The model under review builds one solid part; all positions refer to its coordinate system, in mm. Round coordinates to 2 decimals unless told otherwise and drop trailing zeros. Loops run counter-clockwise (first coordinate to the right, second up) from the corner with the lowest first, then second, coordinate; pieces in that order, holes last. Notation, with made-up numbers: (1.5, -29) - (22.5, -29) arc R29 ccw to (22.5, 5) - close; hole circle Ø5 at (31.25, 65). An arc over 180 degrees is marked (long way). Answer as CSV lines item,"result".
from build123d import *

# Parameters (mm, degrees)
SKETCH1_W                     = 160
SKETCH1_H                     = 100
BASEPLATE_160X100X6_DEPTH     = 6
CORNER_FILLET_R5_R            = 5
M4_ISOLATOR_CLEARANCE_HOLES_D = 4.5


with BuildPart() as part:
    # Sketch1 → BasePlate_160x100x6 (new body)
    with BuildSketch(Plane(origin=(0, 0, 0), x_dir=(1, 0, 0), z_dir=(0, 1, 0))):
        Rectangle(SKETCH1_W, SKETCH1_H)
    extrude(amount=BASEPLATE_160X100X6_DEPTH)

    # Corner_Fillet_R5
    corner_fillet_r5_edges = [part.edges().sort_by_distance(p)[0] for p in [
        (-80, 3, -50),
        (80, 3, -50),
        (80, 3, 50),
        (-80, 3, 50),
    ]]
    fillet(corner_fillet_r5_edges, radius=CORNER_FILLET_R5_R)

    # M4_Isolator_Clearance_Holes (through all)
    with Locations(Plane(origin=(0, 6, 0), x_dir=(1, 0, 0), z_dir=(0, 1, 0))):
        with Locations((-60, 35), (60, 35), (60, -35), (-60, -35)):
            Hole(M4_ISOLATOR_CLEARANCE_HOLES_D / 2)


solid = part.part
1. Draft analysis for pull direction Z (two halves, no side actions). For faces 1 (the face through (61.66, 2.96, -36.52)), 2 (the face through (-80, 3, 1)), 3 (the face through (-79, 3, 48)), state which applies: +Z half, -Z half, draft (parallel to the pull), parting line (faces both ways), or undercut.
Numbers:
face 1,"undercut"
face 2,"draft"
face 3,"+Z half"
2. Take a section at B-B (x = 60). State the section outline as (y, z) points, plus the area to 3 significant figures.
Numbers:
outline,"(0, -50) - (6, -50) - (6, -37.25) - (0, -37.25) - close; (0, -32.75) - (6, -32.75) - (6, 32.75) - (0, 32.75) - close; (0, 37.25) - (6, 37.25) - (6, 50) - (0, 50) - close"
area,"546 mm²"
3. Take a section at A-A (z = -35). State the section outline as (x, y) points, plus the area to 3 significant figures.
Numbers:
outline,"(-80, 0) - (-62.25, 0) - (-62.25, 6) - (-80, 6) - close; (-57.75, 0) - (57.75, 0) - (57.75, 6) - (-57.75, 6) - close; (62.25, 0) - (80, 0) - (80, 6) - (62.25, 6) - close"
area,"906 mm²"
4. Wall thickness on probe 1 along Z at (x, y) = (60, 4.1); probe 2 along X at (y, z) = (4.05, 35): over which ranges is each line inside the solid? List them lowest first.
Numbers:
probe 1,"z = -50 to -37.25, -32.75 to 32.75, 37.25 to 50"
probe 2,"x = -80 to -62.25, -57.75 to 57.75, 62.25 to 80"
